```python
from build123d import *

# Parameters (mm, degrees)
SKETCH1_R           = 8
BOSS_EXTRUDE1_DEPTH = 7
SKETCH2_R           = 17.65
CUT_EXTRUDE1_DEPTH  = 4
SKETCH4_R           = 1.15
CUT_EXTRUDE2_DEPTH  = 3
SKETCH5_R           = 2
CUT_EXTRUDE3_DEPTH  = 2
SKETCH6_R           = 2.5
SKETCH6_R_2         = 1.35
BOSS_EXTRUDE2_DEPTH = 2
SKETCH6_2_R         = 1.35
CUT_EXTRUDE4_DEPTH  = 2
CIRPATTERN3_COUNT   = 4
SKETCH7_W           = 42
SKETCH7_H           = 50
BOSS_EXTRUDE3_DEPTH = 3
FILLET1_R           = 2
CUT_EXTRUDE5_REACH  = 21.445
SKETCH8_W           = 9
SKETCH8_H           = 3


with BuildPart() as part:
    # Sketch1 → Boss-Extrude1 (new body)
    with BuildSketch(Plane.XY):
        with BuildLine():
            Line((-21, 0), (21, 0))
            Line((21, 0), (21, 30))
            ThreePointArc((21, 30), (0, 51), (-21, 30))
            Line((-21, 30), (-21, 0))
        make_face()
        with Locations((0, 30)):
            Circle(SKETCH1_R, mode=Mode.SUBTRACT)
    extrude(amount=BOSS_EXTRUDE1_DEPTH)

    # Sketch2 → Cut-Extrude1 (cut)
    with BuildSketch(Plane(origin=(0, 0, 0), x_dir=(-1, 0, 0), z_dir=(0, 0, -1))):
        with Locations((0, 30)):
            Circle(SKETCH2_R)
    extrude(amount=-CUT_EXTRUDE1_DEPTH, mode=Mode.SUBTRACT)

    # Sketch4 → Cut-Extrude2 (cut)
    with BuildSketch(Plane.XY.offset(7)):
        with Locations((0, 44.5)):
            Circle(SKETCH4_R)
    cut_extrude2 = extrude(amount=-CUT_EXTRUDE2_DEPTH, mode=Mode.SUBTRACT)

    # Sketch5 → Cut-Extrude3 (cut)
    with BuildSketch(Plane.XY.offset(7)):
        with Locations((0, 44.5)):
            Circle(SKETCH5_R)
    cut_extrude3 = extrude(amount=-CUT_EXTRUDE3_DEPTH, mode=Mode.SUBTRACT)

    # Sketch6 → Boss-Extrude2 (add)
    with BuildSketch(Plane.XY.offset(7)):
        with Locations((-13, 43)):
            Circle(SKETCH6_R)
        with Locations((-13, 43)):
            Circle(SKETCH6_R_2, mode=Mode.SUBTRACT)
    boss_extrude2 = extrude(amount=BOSS_EXTRUDE2_DEPTH)

    # Sketch6_2 → Cut-Extrude4 (cut)
    with BuildSketch(Plane.XY.offset(7)):
        with Locations((-13, 43)):
            Circle(SKETCH6_2_R)
    cut_extrude4 = extrude(amount=-CUT_EXTRUDE4_DEPTH, mode=Mode.SUBTRACT)

    # CirPattern3: Cut-Extrude2, Cut-Extrude3, Boss-Extrude2, Cut-Extrude4 ×4 about axis
    cirpattern3_axis = Axis((0, 30, 0), (0, 0, 1))
    for i in range(1, CIRPATTERN3_COUNT):
        add(cut_extrude2.rotate(cirpattern3_axis, i * 360 / CIRPATTERN3_COUNT), mode=Mode.SUBTRACT)
        add(cut_extrude3.rotate(cirpattern3_axis, i * 360 / CIRPATTERN3_COUNT), mode=Mode.SUBTRACT)
        add(boss_extrude2.rotate(cirpattern3_axis, i * 360 / CIRPATTERN3_COUNT))
        add(cut_extrude4.rotate(cirpattern3_axis, i * 360 / CIRPATTERN3_COUNT), mode=Mode.SUBTRACT)

    # Sketch7 → Boss-Extrude3 (add)
    with BuildSketch(Plane.XZ):
        with Locations((0, 3.5)):
            Rectangle(SKETCH7_W, SKETCH7_H)
    extrude(amount=BOSS_EXTRUDE3_DEPTH)

    # Fillet1
    fillet1_edges = [part.edges().sort_by_distance(p)[0] for p in [
        (-21, -1.5, 28.5),
        (-21, -1.5, -21.5),
        (21, -1.5, -21.5),
        (21, -1.5, 28.5),
        (0, 0, 0),
        (0, 0, 7),
    ]]
    fillet(fillet1_edges, radius=FILLET1_R)

    # Sketch8 → Cut-Extrude5 (cut, up to next)
    with BuildSketch(Plane(origin=(22.25, 22.25, 0), x_dir=(0.707106781, -0.707106781, 0), z_dir=(0.707106781, 0.707106781, 0)), mode=Mode.PRIVATE) as cut_extrude5_sk1:
        with Locations((-21.213203436, -4)):
            Rectangle(SKETCH8_W, SKETCH8_H)
    cut_extrude5_tool1 = extrude(cut_extrude5_sk1.sketch, amount=CUT_EXTRUDE5_REACH, mode=Mode.PRIVATE) & part.part
    add(cut_extrude5_tool1.solids().sort_by_distance((7.25, 37.25, 4))[0], mode=Mode.SUBTRACT)


solid = part.part
```
Check sheet for the modelled part. Datum: model origin and axes. Units: mm. A direction names the side the tool comes from. Coordinates: 2 decimals unless noted, no trailing zeros. Loops run counter-clockwise (first coordinate to the right, second up) from the corner with the lowest first, then second, coordinate; pieces in that order, holes last. Notation, with made-up numbers: M -21,-18.75 L 14,-18.75 A19 ccw 14,16.25 Z; hole C 20,-31.75 d9. An arc over 180 degrees is marked long. Answer as a JSON object with one key per item and string values.
1. Depth check by flat-ended pin: P1, Ø6.5, axis at x = 0, y = 44.5, coming from the +Z side; P2, Ø6, axis at y = 42.5, z = 5, coming from the -X side; P3, Ø5, axis at x = 0, y = 15.5, coming from the -Z side. Enter the tip coordinate at first touch or a pass-through.
Outcome:
{"P1": "z = 7", "P2": "x = -18.73", "P3": "z = 4"}
2. Sectioned sample at C-C on y = 7. Record the cut outline in (x, z), and give its area (3 significant figures).
Outcome:
{"outline": "M -21,0 L 21,0 L 21,7 L -21,7 Z", "area": "294 mm²"}
3. Sectioned sample at D-D on z = 11. Record the cut outline in (x, y).
Outcome:
{"outline": "M -21,-3 L 21,-3 L 21,0 L -21,0 Z"}
4. Access from +Z, -Z, +X, -X, +Y, -Y to the whole of each face (thin tool, end or side, straight path). Record for faces 1 (the flat face through (-13, 30, 5)), 2 (the flat face through (11.9, 41.9, 9)), 3 (the flat face through (7.2, 37.3, 4.7)), 4 (the flat face through (0, 11, 0)), 5 (the cylindrical face through (0.29, 0.57, 7.6)).
Outcome:
{"face 1": "+Z", "face 2": "+Z, +X, -X, +Y", "face 3": "-Z", "face 4": "-Z, +X, -X, +Y", "face 5": "+Z, +X, -X"}
5. Release check for a two-part mould opening along Y. For faces 6 (the cylindrical face through (0.249, 16.623, 4.507)), 7 (the flat face through (13, 17, 5)), 8 (the flat face through (0, -3, 4)), 9 (the cylindrical face through (20.4, -1.52, 27.93)) record: pulls with the +Y half, pulls with the -Y half, needs draft (parallel to the pull), parting line crosses it, or undercut.
Outcome:
{"face 6": "undercut", "face 7": "undercut", "face 8": "pulls with the -Y half", "face 9": "needs draft"}
6. Sectioned sample at A-A on x = 0. Count the separate pieces of the cut face and the enclosed holes in it, and give its area (3 significant figures).
Outcome:
{"separate pieces": "4", "enclosed holes": "0", "area": "299 mm²"}
7. Scan lines: L1, parallel to Y at x = 0, z = 6.25; L2, parallel to Z at x = 11, y = 24.5; L3, parallel to Y at x = 5, z = 18. Record each from-to range of solid material in increasing order. Write a range as from..to.
Outcome:
{"L1": "-3..13.5, 17.5..22, 38..42.5, 46.5..51", "L2": "4..7", "L3": "-3..0"}
8. Sectioned sample at B-B on x = -7. Record the cut outline in (y, z).
Outcome:
{"outline": "M -3,-21.5 L 0,-21.5 L 0,-2 A2 cw 2,0 L 13.8,0 L 13.8,4 L 26.13,4 L 26.13,7 L 2,7 A2 cw 0,9 L 0,28.5 L -3,28.5 Z; M 33.87,4 L 46.2,4 L 46.2,0 L 49.8,0 L 49.8,7 L 33.87,7 Z"}
